Autodesk Inventor part; units mm, degrees
ref_plane "Work Plane1" through (0, 0, 12.662) normal (0, 0, -1) x (-1, 0, 0)
ref_plane "YZ Plane" through (0, 0, 0) normal (1, 0, 0) x (0, 1, 0)
ref_plane "XZ Plane" through (0, 0, 0) normal (0, 1, 0) x (-1, 0, 0)
sketch "Sketch1" plane through (0, 0, 0) normal (0, 0, 1) x (1, 0, 0)
  line L0 (0, 103.81) -> (0, 0)
  line L1 (99.04, 103.81) -> (0, 103.81)
  line L2 (99.04, 0) -> (99.04, 103.81)
  circle A0 centre (91.5302, 97.8155) radius 1.6
  circle A1 centre (6.3166, 98.2023) radius 1.6
  circle A2 centre (63.7434, 9.4559) radius 1.6
  line L3 (-2.8877, 39.67) -> (-2.8877, 25.07)
  line L4 (18.04, 39.67) -> (-2.8877, 39.67)
  line L5 (-2.8877, 25.07) -> (18.04, 25.07)
  line L6 (5.99, 20.97) -> (-0.5, 20.97)
  line L7 (-0.5, 20.97) -> (-0.5, 9.286)
  line L8 (-0.5, 9.286) -> (5.99, 9.286)
  line L9 (5.99, 9.286) -> (5.99, 20.97)
  line L10 (18.04, 25.07) -> (18.04, 39.67)
  line L11 (0, 0) -> (99.04, 0)
  line L12 (-2, 105.81) -> (-2, -2)
  line L13 (-2, -2) -> (101.04, -2)
  line L14 (101.04, -2) -> (101.04, 105.81)
  line L15 (101.04, 105.81) -> (-2, 105.81)
  line L16 (-6, 109.81) -> (-6, -6)
  line L17 (-6, -6) -> (105.04, -6)
  line L18 (105.04, -6) -> (105.04, 109.81)
  line L19 (105.04, 109.81) -> (-6, 109.81)
  point P0 (-2, 25.07)
  point P1 (-2, 39.67)
  point P2 (0, 39.67)
  point P3 (0, 9.286)
  point P4 (0, 20.97)
  point P5 (0, 25.07)
  dimension "d0" = 2
  dimension "d1" = 4
extrude "Extrusion1" add sketch "Sketch1" along normal blind 15 contours L0 L4 L12 L15 L14 L13 L5 L6 L7 L8 L11 L2 L1 | L12 L5 L3 L4 | L19 L18 L17 L16
extrude "Extrusion2" add sketch "Sketch1" along normal blind 3 contours L1 L2 L11 L0 L8 L9 L6 L5 L10 L4 | L4 L10 L5 L0 | L0 L5 L12 L4 | L6 L9 L8 L0 | L0 L8 L7 L6 | A0 | A1 | A2
sketch "Sketch2" plane through (0, 0, 3) normal (0, 0, 1) x (1, 0, 0)
  circle A0 centre (63.7434, 9.4559) radius 1.6
  circle A1 centre (91.5302, 97.8155) radius 1.6
  circle A2 centre (6.3166, 98.2023) radius 1.6
  circle A3 centre (6.3166, 98.2023) radius 4
  circle A4 centre (91.5302, 97.8155) radius 4
  circle A5 centre (63.7434, 9.4559) radius 4
  point P0 (0, 0)
  dimension "d8" = 8
  dimension "d9" = 8
  dimension "d10" = 8
extrude "Extrusion4" add sketch "Sketch2" along normal blind 8
ref_plane "Work Plane1" through (0, 0, 12.662) normal (0, 0, -1) x (-1, 0, 0)
sketch "Sketch3" plane through (0, 0, 12.662) normal (0, 0, -1) x (-1, 0, 0)
  line L0 (2, 25.07) -> (2, 39.67)
  line L1 (2, 39.67) -> (6, 39.67)
  line L2 (6, 109.81) -> (6, -6)
  line L3 (0, 20.97) -> (0, 25.07)
  line L4 (6, 39.67) -> (0, 39.67)
  line L5 (0, 39.67) -> (0, 25.07)
  line L6 (0, 25.07) -> (6, 25.07)
  line L7 (6, 25.07) -> (6, 39.67)
  line L8 (0.5, 20.97) -> (0, 20.97)
  line L9 (0.5, 20.97) -> (6, 20.97)
  line L10 (0, 9.286) -> (0.5, 9.286)
  line L11 (0.5, 9.286) -> (6, 9.286)
  line L12 (6, 9.286) -> (6, 20.97)
  line L13 (0.5, 9.286) -> (0.5, 20.97)
  line L14 (0.5, 20.97) -> (0.5, 9.286)
  point P0 (0, 0)
extrude "Extrusion5" cut sketch "Sketch3" against normal blind 8 contours L6 L5 L4 L0 | L0 L1 L2 L6 | L2 L11 L13 L9
fillet "Fillet1" radius 8 4 edges at (-6, 109.81, 7.5) (-6, -6, 7.5) (105.04, -6, 7.5) (105.04, 109.81, 7.5)
sketch "Sketch4" plane through (0, 0, 15) normal (0, 0, 1) x (1, 0, 0)
  line L0 (97.04, 109.81) -> (2, 109.81)
  line L1 (2, 109.81) -> (97.04, 109.81)
  line L2 (0, 103.81) -> (99.04, 103.81)
  line L3 (39.4018, 103.81) -> (59.6382, 103.81)
  line L4 (59.6382, 103.81) -> (59.6382, 109.81)
  line L5 (59.6382, 109.81) -> (39.4018, 109.81)
  line L6 (39.4018, 109.81) -> (39.4018, 103.81)
  line L7 (39.4018, 103.81) -> (59.6382, 109.81) construction
  line L8 (59.6382, 103.81) -> (39.4018, 109.81) construction
  point P0 (0, 0)
  point P1 (49.52, 106.81)
extrude "Extrusion6" cut sketch "Sketch4" against normal up to surface (2.338 mm away)
properties part number "Base"
Could you check a few things on this model? Use its own coordinates, in mm. A direction names the side the tool comes from. Coordinates: 2 decimals unless noted, no trailing zeros. Order: outer loops, then holes, each group sorted by start corner. A loop starts at its lowest first (then second) coordinate and runs counter-clockwise, first axis right, second up. Notation, with made-up numbers: (88, -32) - (145, -32) arc R36 cw to (145, 3) - close; hole circle Ø4 at (72, 77.5). An arc over 180 degrees is marked (long way). Answer in a Markdown table with one row per item. Add a question column.
(1) On a 3-axis mill with a long thin cutter (end or side, diameter ignored), from which of +Z, -Z, +X, -X, +Y, -Y can I reach the whole of each face in a straight line? I mean faces 1 (the face through (-2, 32, 8)), 2 (the face through (49, 53, 0)), 3 (the face through (-3, 15, 12.662)). Say none if no direction works.
(2) If we section it at C-C, the plane x = 48.5: Please give me the cut outline in (y, z).
(3) If we section it at B-B, the plane y = 16: Please give me the cut outline in (x, z).
(4) Will these pins go through, and if not, where does the flat tip stop? pin 1 (2.5 mm diameter, centred on x = 64.5, y = 10, fed in from +Z); pin 2 (6.5 mm diameter, centred on x = -1.5, z = 6, fed in from +Y); pin 3 (5 mm diameter, centred on x = -4, z = 12, fed in from -Y).
(5) I need wall thicknesses on L1, parallel to X at y = 52, z = 9; L2, parallel to Y at x = 57, z = 6.25; L3, parallel to X at y = 36.5, z = 8.75. Which ranges of each line are inside material? Lowest first, please.
(6) If we section it at A-A, the plane z = 8.75: Please give me the cut outline in (x, y).
(7) If we mould it in two halves opening along X, with no side actions, what happens to faces 4 (the face through (-0.2, 82.7, 15)), 5 (the face through (0, 5, 9)), 6 (the face through (102.759, 107.404, 7.605))? For each: released by +X, released by -X, zero draft, split by the parting line, or undercut.
Results are:
| question | item | result |
|---|---|---|
| 1 | face 1 | +Z |
| 1 | face 2 | -Z, +X, -X, +Y, -Y |
| 1 | face 3 | +Z, -X |
| 2 | outline | (-6, 0) - (109.81, 0) - (109.81, 12.66) - (103.81, 12.66) - (103.81, 3) - (0, 3) - (0, 15) - (-6, 15) - close |
| 3 | outline | (-6, 0) - (105.04, 0) - (105.04, 15) - (99.04, 15) - (99.04, 3) - (-0.5, 3) - (-0.5, 12.66) - (-6, 12.66) - close |
| 4 | pin 1 | stops at z = 11 |
| 4 | pin 2 | stops at y = 109.81 |
| 4 | pin 3 | stops at y = -5.19 |
| 5 | L1 | x = -6 to 0, 99.04 to 105.04 |
| 5 | L2 | y = -6 to 0, 103.81 to 109.81 |
| 5 | L3 | x = -6 to -2, 99.04 to 105.04 |
| 6 | outline | (-6, 2) arc R8 ccw to (2, -6) - (97.04, -6) arc R8 ccw to (105.04, 2) - (105.04, 101.81) arc R8 ccw to (97.04, 109.81) - (2, 109.81) arc R8 ccw to (-6, 101.81) - close; circle Ø8 at (6.32, 98.2); circle Ø8 at (63.74, 9.46); circle Ø8 at (91.53, 97.82); hole (-2, 25.07) - (0, 25.07) - (0, 20.97) - (-0.5, 20.97) - (-0.5, 9.29) - (0, 9.29) - (0, 0) - (99.04, 0) - (99.04, 103.81) - (0, 103.81) - (0, 39.67) - (-2, 39.67) - close; hole circle Ø3.2 at (6.32, 98.2); hole circle Ø3.2 at (63.74, 9.46); hole circle Ø3.2 at (91.53, 97.82) |
| 7 | face 4 | zero draft |
| 7 | face 5 | undercut |
| 7 | face 6 | released by +X |
